from build123d import *

# Parameters (mm, degrees)
F0_W     = 9.2964
F0_H     = 18.9992
F1_DEPTH = 0.7874
F2_W     = 9.2964
F2_H     = 13.0048
F3_DEPTH = 2.9718
F4_R     = 0.3937
F5_DEPTH = 25.4
F4_W     = 1.1938
F4_H     = 1.1938
F6_DEPTH = 0.0254
F8_DEPTH = 0.0254


with BuildPart() as f1:
    # F0 (on Top) → F1 (new body)
    with BuildSketch(Plane.XY):
        Rectangle(F0_W, F0_H)
    extrude(amount=F1_DEPTH)

    # F2 (on face) → F3 (join)
    with BuildSketch(Plane.XY.offset(0.7874)):
        Rectangle(F2_W, F2_H)
    extrude(amount=F3_DEPTH)

    # F4 (on face) → F5 (cut)
    with BuildSketch(Plane.XY.offset(0.7874)):
        with BuildLine():
            ThreePointArc((-3.4036, -9.4996), (-3.7973, -9.1059), (-4.191, -9.4996))
            Line((-4.191, -9.4996), (-3.4036, -9.4996))
        make_face()
        with BuildLine():
            ThreePointArc((-1.4986, -9.4996), (-1.8923, -9.1059), (-2.286, -9.4996))
            Line((-2.286, -9.4996), (-1.4986, -9.4996))
        make_face()
        with BuildLine():
            ThreePointArc((0.4064, -9.4996), (0.0127, -9.1059), (-0.381, -9.4996))
            Line((-0.381, -9.4996), (0.4064, -9.4996))
        make_face()
        with BuildLine():
            ThreePointArc((2.3114, -9.4996), (1.9177, -9.1059), (1.524, -9.4996))
            Line((1.524, -9.4996), (2.3114, -9.4996))
        make_face()
        with BuildLine():
            Line((3.429, -9.4996), (4.2164, -9.4996))
            ThreePointArc((4.2164, -9.4996), (3.8227, -9.1059), (3.429, -9.4996))
        make_face()
        with Locations((2.5908, -7.0993)):
            Circle(F4_R)
        with Locations((0, -7.0993)):
            Circle(F4_R)
        with Locations((-2.5908, -7.0993)):
            Circle(F4_R)
        with BuildLine():
            ThreePointArc((-2.3124120602, 7.3776879398), (-2.8691879398, 7.3776879398), (-2.8691879398, 6.8209120602))
            Line((-2.8691879398, 6.8209120602), (-2.3124120602, 7.3776879398))
        make_face()
        with BuildLine():
            Line((-2.3124120602, 7.3776879398), (-2.8691879398, 6.8209120602))
            ThreePointArc((-2.8691879398, 6.8209120602), (-2.4401375327, 6.7355686281), (-2.1971, 7.0993))
            ThreePointArc((-2.1971, 7.0993), (-2.2270686281, 7.2499624673), (-2.3124120602, 7.3776879398))
        make_face()
        with BuildLine():
            ThreePointArc((0.2783879398, 7.3776879398), (-0.2783879398, 7.3776879398), (-0.2783879398, 6.8209120602))
            Line((-0.2783879398, 6.8209120602), (0.2783879398, 7.3776879398))
        make_face()
        with BuildLine():
            Line((0.2783879398, 7.3776879398), (-0.2783879398, 6.8209120602))
            ThreePointArc((-0.2783879398, 6.8209120602), (0.1506624673, 6.7355686281), (0.3937, 7.0993))
            ThreePointArc((0.3937, 7.0993), (0.3637313719, 7.2499624673), (0.2783879398, 7.3776879398))
        make_face()
        with BuildLine():
            ThreePointArc((2.8691879398, 7.3776879398), (2.3124120602, 7.3776879398), (2.3124120602, 6.8209120602))
            Line((2.3124120602, 6.8209120602), (2.8691879398, 7.3776879398))
        make_face()
        with BuildLine():
            Line((2.8691879398, 7.3776879398), (2.3124120602, 6.8209120602))
            ThreePointArc((2.3124120602, 6.8209120602), (2.7414624673, 6.7355686281), (2.9845, 7.0993))
            ThreePointArc((2.9845, 7.0993), (2.9545313719, 7.2499624673), (2.8691879398, 7.3776879398))
        make_face()
        with BuildLine():
            ThreePointArc((-4.191, 9.4996), (-3.7973, 9.1059), (-3.4036, 9.4996))
            Line((-3.4036, 9.4996), (-4.191, 9.4996))
        make_face()
        with BuildLine():
            ThreePointArc((-2.286, 9.4996), (-1.8923, 9.1059), (-1.4986, 9.4996))
            Line((-1.4986, 9.4996), (-2.286, 9.4996))
        make_face()
        with BuildLine():
            Line((0.4064, 9.4996), (-0.381, 9.4996))
            ThreePointArc((-0.381, 9.4996), (0.0127, 9.1059), (0.4064, 9.4996))
        make_face()
        with BuildLine():
            Line((2.3114, 9.4996), (1.524, 9.4996))
            ThreePointArc((1.524, 9.4996), (1.9177, 9.1059), (2.3114, 9.4996))
        make_face()
        with BuildLine():
            Line((4.2164, 9.4996), (3.429, 9.4996))
            ThreePointArc((3.429, 9.4996), (3.8227, 9.1059), (4.2164, 9.4996))
        make_face()
    extrude(amount=-F5_DEPTH, mode=Mode.SUBTRACT)

    # F4 (on face) → F6 (join)
    with BuildSketch(Plane.XY.offset(0.7874)):
        with BuildLine():
            Line((-4.3942, 8.3058), (-3.2004, 8.3058))
            Line((-3.2004, 8.3058), (-3.2004, 9.4996))
            Line((-3.2004, 9.4996), (-3.4036, 9.4996))
            ThreePointArc((-3.4036, 9.4996), (-3.7973, 9.1059), (-4.191, 9.4996))
            Line((-4.191, 9.4996), (-4.3942, 9.4996))
            Line((-4.3942, 9.4996), (-4.3942, 8.3058))
        make_face()
        with BuildLine():
            Line((-1.2954, 9.4996), (-1.4986, 9.4996))
            ThreePointArc((-1.4986, 9.4996), (-1.8923, 9.1059), (-2.286, 9.4996))
            Line((-2.286, 9.4996), (-2.4892, 9.4996))
            Line((-2.4892, 9.4996), (-2.4892, 8.3058))
            Line((-2.4892, 8.3058), (-1.2954, 8.3058))
            Line((-1.2954, 8.3058), (-1.2954, 9.4996))
        make_face()
        with BuildLine():
            Line((-0.381, 9.4996), (-0.5842, 9.4996))
            Line((-0.5842, 9.4996), (-0.5842, 8.3058))
            Line((-0.5842, 8.3058), (0.6096, 8.3058))
            Line((0.6096, 8.3058), (0.6096, 9.4996))
            Line((0.6096, 9.4996), (0.4064, 9.4996))
            ThreePointArc((0.4064, 9.4996), (0.0127, 9.1059), (-0.381, 9.4996))
        make_face()
        with BuildLine():
            Line((1.524, 9.4996), (1.3208, 9.4996))
            Line((1.3208, 9.4996), (1.3208, 8.3058))
            Line((1.3208, 8.3058), (2.5146, 8.3058))
            Line((2.5146, 8.3058), (2.5146, 9.4996))
            Line((2.5146, 9.4996), (2.3114, 9.4996))
            ThreePointArc((2.3114, 9.4996), (1.9177, 9.1059), (1.524, 9.4996))
        make_face()
        with BuildLine():
            Line((3.429, 9.4996), (3.2258, 9.4996))
            Line((3.2258, 9.4996), (3.2258, 8.3058))
            Line((3.2258, 8.3058), (4.4196, 8.3058))
            Line((4.4196, 8.3058), (4.4196, 9.4996))
            Line((4.4196, 9.4996), (4.2164, 9.4996))
            ThreePointArc((4.2164, 9.4996), (3.8227, 9.1059), (3.429, 9.4996))
        make_face()
        with BuildLine():
            Line((-2.4892, -8.3058), (-2.4892, -9.4996))
            Line((-2.4892, -9.4996), (-2.286, -9.4996))
            ThreePointArc((-2.286, -9.4996), (-1.8923, -9.1059), (-1.4986, -9.4996))
            Line((-1.4986, -9.4996), (-1.2954, -9.4996))
            Line((-1.2954, -9.4996), (-1.2954, -8.3058))
            Line((-1.2954, -8.3058), (-2.4892, -8.3058))
        make_face()
        with BuildLine():
            Line((-4.3942, -8.3058), (-4.3942, -9.4996))
            Line((-4.3942, -9.4996), (-4.191, -9.4996))
            ThreePointArc((-4.191, -9.4996), (-3.7973, -9.1059), (-3.4036, -9.4996))
            Line((-3.4036, -9.4996), (-3.2004, -9.4996))
            Line((-3.2004, -9.4996), (-3.2004, -8.3058))
            Line((-3.2004, -8.3058), (-4.3942, -8.3058))
        make_face()
        with BuildLine():
            Line((-0.5842, -8.3058), (-0.5842, -9.4996))
            Line((-0.5842, -9.4996), (-0.381, -9.4996))
            ThreePointArc((-0.381, -9.4996), (0.0127, -9.1059), (0.4064, -9.4996))
            Line((0.4064, -9.4996), (0.6096, -9.4996))
            Line((0.6096, -9.4996), (0.6096, -8.3058))
            Line((0.6096, -8.3058), (-0.5842, -8.3058))
        make_face()
        with BuildLine():
            Line((1.3208, -8.3058), (1.3208, -9.4996))
            Line((1.3208, -9.4996), (1.524, -9.4996))
            ThreePointArc((1.524, -9.4996), (1.9177, -9.1059), (2.3114, -9.4996))
            Line((2.3114, -9.4996), (2.5146, -9.4996))
            Line((2.5146, -9.4996), (2.5146, -8.3058))
            Line((2.5146, -8.3058), (1.3208, -8.3058))
        make_face()
        with BuildLine():
            Line((4.2164, -9.4996), (4.4196, -9.4996))
            Line((4.4196, -9.4996), (4.4196, -8.3058))
            Line((4.4196, -8.3058), (3.2258, -8.3058))
            Line((3.2258, -8.3058), (3.2258, -9.4996))
            Line((3.2258, -9.4996), (3.429, -9.4996))
            ThreePointArc((3.429, -9.4996), (3.8227, -9.1059), (4.2164, -9.4996))
        make_face()
        with Locations((2.5908, -7.0993)):
            Rectangle(F4_W, F4_H)
        with Locations((2.5908, -7.0993)):
            Circle(F4_R, mode=Mode.SUBTRACT)
        with Locations((0, -7.0993)):
            Rectangle(F4_W, F4_H)
        with Locations((0, -7.0993)):
            Circle(F4_R, mode=Mode.SUBTRACT)
        with Locations((-2.5908, -7.0993)):
            Rectangle(F4_W, F4_H)
        with Locations((-2.5908, -7.0993)):
            Circle(F4_R, mode=Mode.SUBTRACT)
        with BuildLine():
            Line((-2.8691879398, 6.8209120602), (-3.1877, 6.5024))
            Line((-3.1877, 6.5024), (-1.9939, 6.5024))
            Line((-1.9939, 6.5024), (-1.9939, 7.6962))
            Line((-1.9939, 7.6962), (-2.3124120602, 7.3776879398))
            ThreePointArc((-2.3124120602, 7.3776879398), (-2.2270686281, 7.2499624673), (-2.1971, 7.0993))
            ThreePointArc((-2.1971, 7.0993), (-2.4401375327, 6.7355686281), (-2.8691879398, 6.8209120602))
        make_face()
        with BuildLine():
            Line((0.5969, 7.6962), (-0.5969, 7.6962))
            Line((-0.5969, 7.6962), (-0.5969, 6.5024))
            Line((-0.5969, 6.5024), (-0.2783879398, 6.8209120602))
            ThreePointArc((-0.2783879398, 6.8209120602), (-0.2783879398, 7.3776879398), (0.2783879398, 7.3776879398))
            Line((0.2783879398, 7.3776879398), (0.5969, 7.6962))
        make_face()
        with BuildLine():
            Line((-0.2783879398, 6.8209120602), (-0.5969, 6.5024))
            Line((-0.5969, 6.5024), (0.5969, 6.5024))
            Line((0.5969, 6.5024), (0.5969, 7.6962))
            Line((0.5969, 7.6962), (0.2783879398, 7.3776879398))
            ThreePointArc((0.2783879398, 7.3776879398), (0.3637313719, 7.2499624673), (0.3937, 7.0993))
            ThreePointArc((0.3937, 7.0993), (0.1506624673, 6.7355686281), (-0.2783879398, 6.8209120602))
        make_face()
        with BuildLine():
            Line((2.3124120602, 6.8209120602), (1.9939, 6.5024))
            Line((1.9939, 6.5024), (3.1877, 6.5024))
            Line((3.1877, 6.5024), (3.1877, 7.6962))
            Line((3.1877, 7.6962), (2.8691879398, 7.3776879398))
            ThreePointArc((2.8691879398, 7.3776879398), (2.9545313719, 7.2499624673), (2.9845, 7.0993))
            ThreePointArc((2.9845, 7.0993), (2.7414624673, 6.7355686281), (2.3124120602, 6.8209120602))
        make_face()
        with BuildLine():
            Line((-3.1877, 7.6962), (-3.1877, 6.5024))
            Line((-3.1877, 6.5024), (-2.8691879398, 6.8209120602))
            ThreePointArc((-2.8691879398, 6.8209120602), (-2.8691879398, 7.3776879398), (-2.3124120602, 7.3776879398))
            Line((-2.3124120602, 7.3776879398), (-1.9939, 7.6962))
            Line((-1.9939, 7.6962), (-3.1877, 7.6962))
        make_face()
        with BuildLine():
            Line((1.9939, 7.6962), (1.9939, 6.5024))
            Line((1.9939, 6.5024), (2.3124120602, 6.8209120602))
            ThreePointArc((2.3124120602, 6.8209120602), (2.3124120602, 7.3776879398), (2.8691879398, 7.3776879398))
            Line((2.8691879398, 7.3776879398), (3.1877, 7.6962))
            Line((3.1877, 7.6962), (1.9939, 7.6962))
        make_face()
    extrude(amount=F6_DEPTH)

    # F7 (on face) → F8 (cut)
    with BuildSketch(Plane.XY.offset(3.7592)):
        Polygon((-1.6337567293, 5.08), (-2.2369401238, 4.5738690361), (-3.8328201964, -4.4768166055), (-3.3266892325, -5.08), (1.6337567293, -5.08), (2.2369401238, -4.5738690361), (3.8328201964, 4.4768166055), (3.3266892325, 5.08), align=None)
        Polygon((-0.6995260408, -1.6999813781), (-1.1566746545, -4.2926), (-2.496976666, -4.2926), align=None, mode=Mode.SUBTRACT)
        Polygon((-0.7520136768, -0.3937), (-2.8458346333, -3.4137992041), (-2.3133096593, -0.3937), align=None, mode=Mode.SUBTRACT)
        Polygon((0.097116606, -1.716452297), (0.8590653228, -4.2926), (-0.3571277403, -4.2926), align=None, mode=Mode.SUBTRACT)
        Polygon((2.1744697946, -0.3937), (1.5591465579, -3.8833714858), (0.5270043762, -0.3937), align=None, mode=Mode.SUBTRACT)
        Polygon((-2.1744697946, 0.3937), (-1.5591465579, 3.8833714858), (-0.5270043762, 0.3937), align=None, mode=Mode.SUBTRACT)
        Polygon((-0.8590653228, 4.2926), (0.3571277403, 4.2926), (-0.097116606, 1.716452297), align=None, mode=Mode.SUBTRACT)
        Polygon((2.8458346333, 3.4137992041), (2.3133096593, 0.3937), (0.7520136768, 0.3937), align=None, mode=Mode.SUBTRACT)
        Polygon((1.1566746545, 4.2926), (2.496976666, 4.2926), (0.6995260408, 1.6999813781), align=None, mode=Mode.SUBTRACT)
    extrude(amount=-F8_DEPTH, mode=Mode.SUBTRACT)


solid = f1.part
Read the model definition and answer for the solid it produces. Units are mm, in the model's axes. A direction names the side the tool comes from. Give positions to 0.01 mm unless a question says otherwise; leave off trailing zeros. Loops run counter-clockwise (first coordinate to the right, second up) from the corner with the lowest first, then second, coordinate; pieces in that order, holes last. Notation, with made-up numbers: (72, 16) -> (111, 16) arc R12 ccw to (111, 24) -> close; hole circle Ø2 at (59, 72.25). An arc over 180 degrees is marked (long way). Use a Markdown table: item, result.
Q1. A tool of negligible diameter and unlimited length cuts with its end or side. For faces 1 (the face through (-4.648, 0, 2)), 2 (the face through (-3.8, -8.8, 0.813)), 3 (the face through (0, 8.8, 0.813)), from which of +Z, -Z, +X, -X, +Y, -Y can it reach the whole face along a straight path? Write none if from no direction.
Solved:
| item | result |
|---|---|
| face 1 | +Z, -Z, -X, +Y, -Y |
| face 2 | +Z, +X, -X, -Y |
| face 3 | +Z, +X, -X, +Y |
Q2. Find the intervals of material crossed by line 1 along Y through (x, z) = (0, 0.35); line 2 along Y through (x, z) = (-2, 2.9); line 3 along Y through (x, z) = (2.75, 0.7), in increasing order.
Solved:
| item | result |
|---|---|
| line 1 | y = -9.11 to -7.49, -6.71 to 6.71, 7.49 to 9.11 |
| line 2 | y = -6.5 to 6.5 |
| line 3 | y = -9.5 to -7.46, -6.74 to 6.74, 7.46 to 9.5 |
Q3. Section A-A, the plane z = 1.85 is taken. Determine the outline of the cut face in (x, y), then the cut area to 3 significant figures.
Solved:
| item | result |
|---|---|
| outline | (-4.65, -6.5) -> (4.65, -6.5) -> (4.65, 6.5) -> (-4.65, 6.5) -> close |
| area | 121 mm^2 |
Q4. Determine the mould class of faces 4 (the face through (0, 8, 0.787)), 5 (the face through (3.8, -8.8, 0.813)), 6 (the face through (1, -9.5, 0.4)) for opening direction Y: pulls with the +Y half, pulls with the -Y half, needs draft (parallel to the pull), parting line crosses it, or undercut.
Solved:
| item | result |
|---|---|
| face 4 | undercut |
| face 5 | needs draft |
| face 6 | pulls with the -Y half |
Q5. Each of these flat-tipped pins is pushed along its axis until it touches: pin 1 (1 mm diameter, centred on x = 3.5, z = 2.5, fed in from -Y); pin 2 (1.5 mm diameter, centred on x = 1, z = 1.5, fed in from +Y); pin 3 (1.5 mm diameter, centred on x = -2.5, z = 3, fed in from +Y); pin 4 (1.3 mm diameter, centred on x = 3.5, y = 9, fed in from +Z). Where does it stop, or does it pass through?
Solved:
| item | result |
|---|---|
| pin 1 | stops at y = -6.5 |
| pin 2 | stops at y = 9.5 |
| pin 3 | stops at y = 6.5 |
| pin 4 | stops at z = 0.81 |
